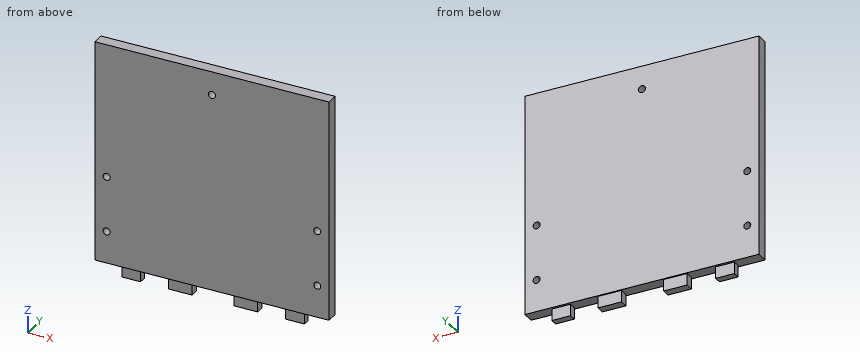
from build123d import *

# Parameters (mm, degrees)
SKETCH1_W           = 200
SKETCH1_H           = 190
BOSS_EXTRUDE1_DEPTH = 10
SKETCH2_W           = 16
SKETCH2_H           = 6
SKETCH2_W_2         = 20
SKETCH2_H_2         = 7
BOSS_EXTRUDE2_DEPTH = 10
SKETCH3_R           = 3
CUT_EXTRUDE1_DEPTH  = 10
SKETCH4_R           = 3
CUT_EXTRUDE2_DEPTH  = 10


with BuildPart() as part:
    # Sketch1 → Boss-Extrude1 (new body)
    with BuildSketch(Plane(origin=(0, 0, 0), x_dir=(1, 0, 0), z_dir=(0, 1, 0))):
        with Locations((100, 95)):
            Rectangle(SKETCH1_W, SKETCH1_H)
    extrude(amount=BOSS_EXTRUDE1_DEPTH)

    # Sketch2 → Boss-Extrude2 (add)
    with BuildSketch(Plane(origin=(0, 0, -190), x_dir=(-1, 0, 0), z_dir=(0, 0, -1))):
        with Locations((-30, 5)):
            Rectangle(SKETCH2_W, SKETCH2_H)
        with Locations((-170, 5)):
            Rectangle(SKETCH2_W, SKETCH2_H)
        with Locations((-128, 5.5)):
            Rectangle(SKETCH2_W_2, SKETCH2_H_2)
        with Locations((-72, 5.5)):
            Rectangle(SKETCH2_W_2, SKETCH2_H_2)
    extrude(amount=BOSS_EXTRUDE2_DEPTH)

    # Sketch3 → Cut-Extrude1 (cut)
    with BuildSketch(Plane(origin=(0, 10, 0), x_dir=(1, 0, 0), z_dir=(0, 1, 0))):
        with Locations(Location((190, 162.5, 0), (0, 0, 270))):
            Circle(SKETCH3_R)
        with Locations(Location((190, 115, 0), (0, 0, 270))):
            Circle(SKETCH3_R)
        with Locations(Location((10, 162.5, 0), (0, 0, 90))):
            Circle(SKETCH3_R)
        with Locations(Location((10, 115, 0), (0, 0, 90))):
            Circle(SKETCH3_R)
    extrude(amount=-CUT_EXTRUDE1_DEPTH, mode=Mode.SUBTRACT)

    # Sketch4 → Cut-Extrude2 (cut)
    with BuildSketch(Plane(origin=(0, 10, 0), x_dir=(1, 0, 0), z_dir=(0, 1, 0))):
        with Locations(Location((100, 20, 0), (0, 0, 270))):
            Circle(SKETCH4_R)
    extrude(amount=-CUT_EXTRUDE2_DEPTH, mode=Mode.SUBTRACT)


solid = part.part
Verification items for the finished model (mm, model axes). Coordinates: 2 decimals unless noted, no trailing zeros. Loops run counter-clockwise (first coordinate to the right, second up) from the corner with the lowest first, then second, coordinate; pieces in that order, holes last. Notation, with made-up numbers: (36.25, 65.5) -> (87.25, 65.5) arc R24 ccw to (87.25, 94.5) -> close; hole circle Ø2 at (26.5, -5.5). An arc over 180 degrees is marked (long way). Answer as a JSON object with one key per item and string values. Group by question number.
Item 1: Sectioned sample at D-D on x = 190. Record the boundary of the cut face in (y, z), plus the area to 3 significant figures.
Item 2: Sectioned sample at B-B on z = -162.5. Record the boundary of the cut face in (x, y).
Item 3: Depth check by flat-ended pin: pin 1 (3 mm diameter, centred on x = 124.5, z = -193.5, fed in from +Y); pin 2 (3 mm diameter, centred on x = 116, y = 6.5, fed in from -Z); pin 3 (5.5 mm diameter, centred on y = 4.5, z = -196.5, fed in from +X); pin 4 (5.5 mm diameter, centred on x = 190, z = -162.5, fed in from -Y). Enter the tip coordinate at first touch or a pass-through.
Item 4: Sectioned sample at A-A on x = 100. Record the boundary of the cut face in (y, z), plus the area to 3 significant figures.
Item 5: Scan lines: probe 1 along Z at (x, y) = (10, 2); probe 2 along X at (y, z) = (7.75, -115); probe 3 along Z at (x, y) = (144, 4.5). Record each from-to range of solid material in increasing order.
Item 6: Sectioned sample at C-C on y = 5. Record the boundary of the cut face in (x, z), plus the area to 3 significant figures.
Evaluation:
{
 "1": {"outline": "(0, -190) -> (10, -190) -> (10, -165.5) -> (0, -165.5) -> close; (0, -159.5) -> (10, -159.5) -> (10, -118) -> (0, -118) -> close; (0, -112) -> (10, -112) -> (10, 0) -> (0, 0) -> close", "area": "1,780 mm²"},
 "2": {"outline": "(0, 0) -> (7, 0) -> (7, 10) -> (0, 10) -> close; (13, 0) -> (187, 0) -> (187, 10) -> (13, 10) -> close; (193, 0) -> (200, 0) -> (200, 10) -> (193, 10) -> close"},
 "3": {"pin 1": "stops at y = 9", "pin 2": "stops at z = -190", "pin 3": "stops at x = 178", "pin 4": "passes through"},
 "4": {"outline": "(0, -190) -> (10, -190) -> (10, -23) -> (0, -23) -> close; (0, -17) -> (10, -17) -> (10, 0) -> (0, 0) -> close", "area": "1,840 mm²"},
 "5": {"probe 1": "z = -190 to -165.5, -159.5 to -118, -112 to 0", "probe 2": "x = 0 to 7, 13 to 187, 193 to 200", "probe 3": "z = -190 to 0"},
 "6": {"outline": "(0, -190) -> (22, -190) -> (22, -200) -> (38, -200) -> (38, -190) -> (62, -190) -> (62, -200) -> (82, -200) -> (82, -190) -> (118, -190) -> (118, -200) -> (138, -200) -> (138, -190) -> (162, -190) -> (162, -200) -> (178, -200) -> (178, -190) -> (200, -190) -> (200, 0) -> (0, 0) -> close; hole circle Ø6 at (10, -162.5); hole circle Ø6 at (10, -115); hole circle Ø6 at (100, -20); hole circle Ø6 at (190, -162.5); hole circle Ø6 at (190, -115)", "area": "38,600 mm²"}
}
